from build123d import *

# Parameters (mm, degrees)
SKETCH1_W           = 127
SKETCH1_H           = 241.3
BOSS_EXTRUDE1_DEPTH = 38.1
CUT_EXTRUDE1_REACH  = 254.408
SKETCH3_W           = 25.146
SKETCH3_H           = 81.026
CUT_EXTRUDE2_DEPTH  = 37.5875
SKETCH4_W           = 56.27
SKETCH4_H           = 8.636
CUT_EXTRUDE3_DEPTH  = 61.9125
SKETCH5_W           = 127
SKETCH5_H           = 156.845
CUT_EXTRUDE4_DEPTH  = 22.4917
CUT_EXTRUDE5_REACH  = 148.538
SKETCH6_R           = 2.38125
SKETCH7_W           = 12.7
SKETCH7_H           = 101.6
CUT_EXTRUDE6_DEPTH  = 12.7


with BuildPart() as part:
    # Sketch1 → Boss-Extrude1 (new, symmetric)
    with BuildSketch(Plane.XY):
        Rectangle(SKETCH1_W, SKETCH1_H)
    extrude(amount=BOSS_EXTRUDE1_DEPTH, both=True)

    # Sketch2 → Cut-Extrude1 (cut, up to next)
    with BuildSketch(Plane(origin=(0, 120.65, 0), x_dir=(1, 0, 0), z_dir=(0, 1, 0)), mode=Mode.PRIVATE) as cut_extrude1_sk1:
        with BuildLine():
            Line((-3.96875, -38.1), (-3.96875, -34.13125))
            ThreePointArc((-3.96875, -34.13125), (0, -30.1625), (3.96875, -34.13125))
            Line((3.96875, -34.13125), (3.96875, -38.1))
            Line((3.96875, -38.1), (-3.96875, -38.1))
        make_face()
    cut_extrude1_tool1 = extrude(cut_extrude1_sk1.sketch, amount=-CUT_EXTRUDE1_REACH, mode=Mode.PRIVATE) & part.part
    add(cut_extrude1_tool1.solids().sort_by_distance((0, 120.65, 34.501732))[0], mode=Mode.SUBTRACT)

    # Sketch3 → Cut-Extrude2 (cut)
    with BuildSketch(Plane(origin=(0, 0, -38.1), x_dir=(-1, 0, 0), z_dir=(0, 0, -1))):
        Polygon((-37.614075, 78.105), (-37.614075, 57.8612), (-37.614075, 39.878), (-37.614075, 31.75), (-37.614075, 1.905), (-23.644075, 1.905), (-23.644075, 29.845), (-17.167075, 29.845), (-17.167075, 1.905), (1.120925, 1.905), (1.120925, 29.845), (4.295925, 29.845), (4.295925, 78.105), (-13.877775, 78.105), (-13.877775, 96.139), (-25.676075, 96.139), (-25.676075, 78.105), align=None)
        with Locations((32.108925, 42.418)):
            Rectangle(SKETCH3_W, SKETCH3_H)
    extrude(amount=-CUT_EXTRUDE2_DEPTH, mode=Mode.SUBTRACT)

    # Sketch4 → Cut-Extrude3 (cut)
    with BuildSketch(Plane(origin=(0, 0, -38.1), x_dir=(-1, 0, 0), z_dir=(0, 0, -1))):
        with Locations((-15.276925, 97.917)):
            Rectangle(SKETCH4_W, SKETCH4_H)
    extrude(amount=-CUT_EXTRUDE3_DEPTH, mode=Mode.SUBTRACT)

    # Sketch5 → Cut-Extrude4 (cut)
    with BuildSketch(Plane(origin=(0, 0, -38.1), x_dir=(-1, 0, 0), z_dir=(0, 0, -1))):
        with Locations((0, 42.2275)):
            Rectangle(SKETCH5_W, SKETCH5_H)
    extrude(amount=-CUT_EXTRUDE4_DEPTH, mode=Mode.SUBTRACT)

    # Sketch6 → Cut-Extrude5 (cut, up to next)
    with BuildSketch(Plane(origin=(0, 0, -15.6083), x_dir=(-1, 0, 0), z_dir=(0, 0, -1)), mode=Mode.PRIVATE) as cut_extrude5_sk1:
        with Locations((-50.8, -24.28875)):
            Circle(SKETCH6_R)
    cut_extrude5_tool1 = extrude(cut_extrude5_sk1.sketch, amount=-CUT_EXTRUDE5_REACH, mode=Mode.PRIVATE) & part.part
    # Sketch6 → Cut-Extrude5 (cut, up to next)
    with BuildSketch(Plane(origin=(0, 0, -15.6083), x_dir=(-1, 0, 0), z_dir=(0, 0, -1)), mode=Mode.PRIVATE) as cut_extrude5_sk2:
        with Locations((50.8, 107.95)):
            Circle(SKETCH6_R)
    cut_extrude5_tool2 = extrude(cut_extrude5_sk2.sketch, amount=-CUT_EXTRUDE5_REACH, mode=Mode.PRIVATE) & part.part
    # Sketch6 → Cut-Extrude5 (cut, up to next)
    with BuildSketch(Plane(origin=(0, 0, -15.6083), x_dir=(-1, 0, 0), z_dir=(0, 0, -1)), mode=Mode.PRIVATE) as cut_extrude5_sk3:
        with Locations((50.8, -24.28875)):
            Circle(SKETCH6_R)
    cut_extrude5_tool3 = extrude(cut_extrude5_sk3.sketch, amount=-CUT_EXTRUDE5_REACH, mode=Mode.PRIVATE) & part.part
    # Sketch6 → Cut-Extrude5 (cut, up to next)
    with BuildSketch(Plane(origin=(0, 0, -15.6083), x_dir=(-1, 0, 0), z_dir=(0, 0, -1)), mode=Mode.PRIVATE) as cut_extrude5_sk4:
        with Locations((-50.8, 107.95)):
            Circle(SKETCH6_R)
    cut_extrude5_tool4 = extrude(cut_extrude5_sk4.sketch, amount=-CUT_EXTRUDE5_REACH, mode=Mode.PRIVATE) & part.part
    add(cut_extrude5_tool1.solids().sort_by_distance((50.8, -24.28875, -15.6083))[0], mode=Mode.SUBTRACT)
    add(cut_extrude5_tool2.solids().sort_by_distance((-50.8, 107.95, -15.6083))[0], mode=Mode.SUBTRACT)
    add(cut_extrude5_tool3.solids().sort_by_distance((-50.8, -24.28875, -15.6083))[0], mode=Mode.SUBTRACT)
    add(cut_extrude5_tool4.solids().sort_by_distance((50.8, 107.95, -15.6083))[0], mode=Mode.SUBTRACT)

    # Sketch7 → Cut-Extrude6 (cut)
    with BuildSketch(Plane(origin=(63.5, 0, 0), x_dir=(0, 0, -1), z_dir=(1, 0, 0))):
        with Locations((-11.24585, 0)):
            Rectangle(SKETCH7_W, SKETCH7_H)
    extrude(amount=-CUT_EXTRUDE6_DEPTH, mode=Mode.SUBTRACT)


solid = part.part
Here's how the part is built. I have some questions about the finished solid (model axes, mm). A direction names the side the tool comes from. Round coordinates to 2 decimals unless told otherwise and drop trailing zeros. Order: outer loops, then holes, each group sorted by start corner. A loop starts at its lowest first (then second) coordinate and runs counter-clockwise, first axis right, second up. Notation, with made-up numbers: M 32.25,-32.75 L 65.25,-32.75 A25 ccw 65.25,2.25 Z; hole C 61.5,49.25 d1. An arc over 180 degrees is marked long. Return JSON: item names as keys, results as strings. Group by question number.
1. I'm going to push flat-ended pins straight in: pin 1 Ø10 at (y, z) = (23.5, 10.5) entering from +X; pin 2 Ø6 at (x, y) = (36.5, 67) entering from -Z; pin 3 Ø7.5 at (x, y) = (-28.5, 57) entering from -Z. Where does each tip first touch, or does it pass through?
2. If we section it at C-C on y = 16.5: List the corners of the cut face in (x, z) for me.
3. If we mould it in two halves opening along Z, with no side actions, what happens to faces 1 (the face through (32, 78.105, -8)), 2 (the face through (50.8, 15, 11)), 3 (the face through (-13, 43, -15.608))? For each: pulls with the +Z half, pulls with the -Z half, needs draft (parallel to the pull), parting line crosses it, or undercut.
4. Please list where these lines run through material, in increasing order: probe 1 along Y at (x, z) = (50.8, 18); probe 2 along Z at (x, y) = (54.5, -14); probe 3 along Y at (x, z) = (50, 16).
5. On a 3-axis mill with a long thin cutter (end or side, diameter ignored), from which of +Z, -Z, +X, -X, +Y, -Y can I reach the whole of each face in a straight line? I mean faces 4 (the face through (48.53, -23.57, 10.87)), 5 (the face through (8, 1.905, -8)), 6 (the face through (57, 50.8, 11)). Say none if no direction works.
6. If we section it at B-B on x = -50.8: State how many separate pieces and enclosed holes the cut face has, then the cut area to 3 significant figures.
7. If we section it at A-A on y = 107.95: List the corners of the cut face in (x, z) for me.
Reply:
{
 "1": {"pin 1": "x = 50.8", "pin 2": "z = -15.61", "pin 3": "z = -0.51"},
 "2": {"outline": "M -63.5,-15.61 L -44.68,-15.61 L -44.68,-0.51 L -19.54,-0.51 L -19.54,-15.61 L -1.12,-15.61 L -1.12,-0.51 L 17.17,-0.51 L 17.17,-15.61 L 23.64,-15.61 L 23.64,-0.51 L 37.61,-0.51 L 37.61,-15.61 L 63.5,-15.61 L 63.5,4.9 L 50.8,4.9 L 50.8,17.6 L 63.5,17.6 L 63.5,38.1 L 3.97,38.1 L 3.97,34.13 A3.97 cw -3.97,34.13 L -3.97,38.1 L -63.5,38.1 Z"},
 "3": {"face 1": "needs draft", "face 2": "undercut", "face 3": "pulls with the -Z half"},
 "4": {"probe 1": "-120.65 to -26.67, -21.91 to 105.57, 110.33 to 120.65", "probe 2": "-15.61 to 4.9, 17.6 to 38.1", "probe 3": "-120.65 to -26.53, -22.05 to 105.71, 110.19 to 120.65"},
 "5": {"face 4": "+Z, -Z", "face 5": "-Z", "face 6": "+X"},
 "6": {"separate pieces": "3", "enclosed holes": "0", "area": "14,300 mm^2"},
 "7": {"outline": "M -63.5,-15.61 L -53.18,-15.61 L -53.18,38.1 L -63.5,38.1 Z; M -48.42,-15.61 L 48.42,-15.61 L 48.42,38.1 L 3.97,38.1 L 3.97,34.13 A3.97 cw -3.97,34.13 L -3.97,38.1 L -48.42,38.1 Z; M 53.18,-15.61 L 63.5,-15.61 L 63.5,38.1 L 53.18,38.1 Z"}
}
